```python
from build123d import *

# Parameters (mm, degrees)
SKETCH2_R                                = 100
BOSS_EXTRUDE1_DEPTH                      = 30
BOSS_EXTRUDE2_DEPTH                      = 28
BOSS_EXTRUDE3_DEPTH                      = 50
CBORE_FOR_1_4_HEX_HEAD_BOLT1_D           = 6.7564
CBORE_FOR_1_4_HEX_HEAD_BOLT1_CBORE_D     = 19.05
CBORE_FOR_1_4_HEX_HEAD_BOLT1_CBORE_DEPTH = 4.7752


with BuildPart() as part:
    # Sketch2 → Boss-Extrude1 (new body)
    with BuildSketch(Plane(origin=(0, 0, 0), x_dir=(1, 0, 0), z_dir=(0, 1, 0))):
        with Locations(Location((0, 0, 0), (0, 0, 270))):
            Circle(SKETCH2_R)
    extrude(amount=BOSS_EXTRUDE1_DEPTH)

    # Sketch3 → Boss-Extrude2 (add)
    with BuildSketch(Plane(origin=(0, 30, 0), x_dir=(1, 0, 0), z_dir=(0, 1, 0))):
        with BuildLine():
            ThreePointArc((20, 97.979589711), (0, 100), (-20, 97.979589711))
            Line((-20, 97.979589711), (-20, 69.686799324))
            ThreePointArc((-20, 69.686799324), (-51.265241636, 51.265241636), (-69.686799324, 20))
            Line((-69.686799324, 20), (-97.979589711, 20))
            ThreePointArc((-97.979589711, 20), (-100, 0), (-97.979589711, -20))
            Line((-97.979589711, -20), (-69.686799324, -20))
            ThreePointArc((-69.686799324, -20), (-51.265241636, -51.265241636), (-20, -69.686799324))
            Line((-20, -69.686799324), (-20, -97.979589711))
            ThreePointArc((-20, -97.979589711), (0, -100), (20, -97.979589711))
            Line((20, -97.979589711), (20, -69.686799324))
            ThreePointArc((20, -69.686799324), (51.265241636, -51.265241636), (69.686799324, -20))
            Line((69.686799324, -20), (97.979589711, -20))
            ThreePointArc((97.979589711, -20), (99.493615301, -10.050896201), (100, 0))
            ThreePointArc((100, 0), (99.493615301, 10.050896201), (97.979589711, 20))
            Line((97.979589711, 20), (69.686799324, 20))
            ThreePointArc((69.686799324, 20), (51.265241636, 51.265241636), (20, 69.686799324))
            Line((20, 69.686799324), (20, 97.979589711))
        make_face()
    extrude(amount=BOSS_EXTRUDE2_DEPTH)

    # Sketch4 → Boss-Extrude3 (add)
    with BuildSketch(Plane(origin=(0, 58, 0), x_dir=(1, 0, 0), z_dir=(0, 1, 0))):
        with BuildLine():
            Line((-9.722222222, 23.0321166), (-47.916666667, 6.90963498))
            ThreePointArc((-47.916666667, 6.90963498), (-52.5, 0), (-47.916666667, -6.90963498))
            Line((-47.916666667, -6.90963498), (-9.722222222, -23.0321166))
            ThreePointArc((-9.722222222, -23.0321166), (0, -25), (9.722222222, -23.0321166))
            Line((9.722222222, -23.0321166), (47.916666667, -6.90963498))
            ThreePointArc((47.916666667, -6.90963498), (52.5, 0), (47.916666667, 6.90963498))
            Line((47.916666667, 6.90963498), (9.722222222, 23.0321166))
            ThreePointArc((9.722222222, 23.0321166), (0, 25), (-9.722222222, 23.0321166))
        make_face()
    extrude(amount=BOSS_EXTRUDE3_DEPTH)

    # CBORE for 1/4 Hex Head Bolt1 (through all)
    with Locations(Plane(origin=(-82.955537588, 58, 0.659036268), x_dir=(0, 0, 1), z_dir=(0, 1, 0))):
        with Locations((0, 0), (0.670356689, 164.496030798)):
            CounterBoreHole(CBORE_FOR_1_4_HEX_HEAD_BOLT1_D / 2, CBORE_FOR_1_4_HEX_HEAD_BOLT1_CBORE_D / 2, CBORE_FOR_1_4_HEX_HEAD_BOLT1_CBORE_DEPTH)

    # Sketch8 → 1/4 (0.25) Diameter Hole1 (revolve, cut)
    with BuildSketch(Plane(origin=(-45, 108, 0), x_dir=(0, 0, 1), z_dir=(1, 0, 0))):
        Polygon((0, 0), (0, 1.957732465), (3.175, 0.05), (3.175, 0), align=None)
    f_1_4_0_25_diameter_hole1 = revolve(axis=Axis((-45, 114.35, 0), (0, -1, 0)), mode=Mode.SUBTRACT)

    # Mirror1: 1/4 (0.25) Diameter Hole1 across plane
    add(f_1_4_0_25_diameter_hole1.mirror(Plane(origin=(0, 0, 0), x_dir=(0, 0, 1), z_dir=(1, 0, 0))), mode=Mode.SUBTRACT)

    # Sketch9 → Cut-Revolve1 (revolve, cut)
    with BuildSketch(Plane.XY, mode=Mode.PRIVATE) as cut_revolve1_sk:
        with BuildLine():
            Line((0, 108), (-22, 108))
            Line((-22, 108), (-22, 100))
            Line((-22, 100), (-12.5, 100))
            Line((-12.5, 100), (-12.5, 62))
            Line((-12.5, 62), (-5, 62))
            Line((-5, 62), (-5, 49))
            Line((-5, 49), (-15.789877929, 49))
            ThreePointArc((-15.789877929, 49), (-24.423738044, 45.423738044), (-28, 36.789877929))
            Line((-28, 36.789877929), (-28, 25))
            Line((-28, 25), (-40, 25))
            Line((-40, 25), (-40, 0))
            Line((-40, 0), (0, 0))
            Line((0, 0), (0, 108))
        make_face()
    revolve(cut_revolve1_sk.sketch.rotate(Axis((0, 0, 0), (0, 1, 0)), 270), axis=Axis((0, 0, 0), (0, 1, 0)), mode=Mode.SUBTRACT)


solid = part.part
```
CAD build for the part. Positions are in the model's coordinates, mm. A direction names the side the tool comes from. Coordinates: 2 decimals unless noted, no trailing zeros. Order: outer loops, then holes, each group sorted by start corner. A loop starts at its lowest first (then second) coordinate and runs counter-clockwise, first axis right, second up.
(1) Pin check, flat tips, straight feed: pin 1 Ø5.5 at (x, z) = (-82.96, 0.66) entering from +Y; pin 2 Ø3 at (x, z) = (9, -5) entering from +Y; pin 3 Ø23.5 at (x, z) = (-74, -45) entering from +Y; pin 4 Ø6 at (x, y) = (-54.5, 27) entering from +Z. Stop position of each tip, or through.
Solution:
pin 1: passes through
pin 2: stops at y = 62
pin 3: stops at y = 30
pin 4: stops at z = 85.72
(2) Drill centre lines: L1, parallel to Y at x = 12, z = -39; L2, parallel to Y at x = -63, z = 61; L3, parallel to Z at x = 1, y = 5 (1 decimal). Where is each one in solid material? Low to high.
Solution:
L1: y = 0 to 58
L2: y = 0 to 30
L3: z = -100 to -40, 40 to 100
(3) Saw through at B-B, the plane z = -74. Write the cut outline in (x, y), and give its area (3 significant figures).
Solution:
outline: (-67.26, 0) - (67.26, 0) - (67.26, 30) - (20, 30) - (20, 58) - (-20, 58) - (-20, 30) - (-67.26, 30) - close
area: 5,160 mm2
(4) Which spindle directions (+Z, -Z, +X, -X, +Y, -Y) get a long thin tool onto all of the face, cutting with end or side? Do faces 5 (the face through (-20, 44, 84)), 6 (the face through (60, 30, 58)), 7 (the face through (-3.755, 80.734, -11.923)), 8 (the face through (29.087, 82.65, -14.858)), 9 (the face through (-50.9, 43.8, -51.63)). Say none if no direction does.
Solution:
face 5: +Z, -X, +Y
face 6: +Z, +X, +Y
face 7: +Y
face 8: -Z, +X, +Y
face 9: -Z, -X, +Y
(5) Saw through at D-D, the plane y = 9.5. Write the cut outline in (x, z).
Solution:
outline: circle Ø200 at (0, 0); hole circle Ø6.76 at (-82.96, 0.66); hole circle Ø80 at (0, 0); hole circle Ø6.76 at (81.54, 1.33)
(6) Saw through at C-C, the plane x = 67. Write the cut outline in (y, z), and give its area (3 significant figures).
Solution:
outline: (0, -74.24) - (30, -74.24) - (30, -27.7) - (58, -27.7) - (58, 27.7) - (30, 27.7) - (30, 74.24) - (0, 74.24) - close
area: 6,010 mm2
(7) Saw through at A-A, the plane y = 45. Write the cut outline in (x, z), and give its area (3 significant figures).
Solution:
outline: (-97.98, -20) - (-69.69, -20) arc R72.5 ccw to (-20, -69.69) - (-20, -97.98) arc R100 ccw to (20, -97.98) - (20, -69.69) arc R72.5 ccw to (69.69, -20) - (97.98, -20) arc R100 ccw to (97.98, 20) - (69.69, 20) arc R72.5 ccw to (20, 69.69) - (20, 97.98) arc R100 ccw to (-20, 97.98) - (-20, 69.69) arc R72.5 ccw to (-69.69, 20) - (-97.98, 20) arc R100 ccw to start; hole circle Ø6.76 at (-82.96, 0.66); hole circle Ø49.66 at (0, 0); hole circle Ø6.76 at (81.54, 1.33)
area: 18,900 mm2
(8) Mould opens along X. For faces 1 (the face through (0, 83, 25)), 2 (the face through (50.9, 43.8, 51.63)), 3 (the face through (45.547, 106.374, -0.072)), 4 (the face through (84, 44, -20)) say: released by +X, released by -X, zero draft, split by the parting line, or undercut.
Solution:
face 1: split by the parting line
face 2: released by +X
face 3: undercut
face 4: zero draft
